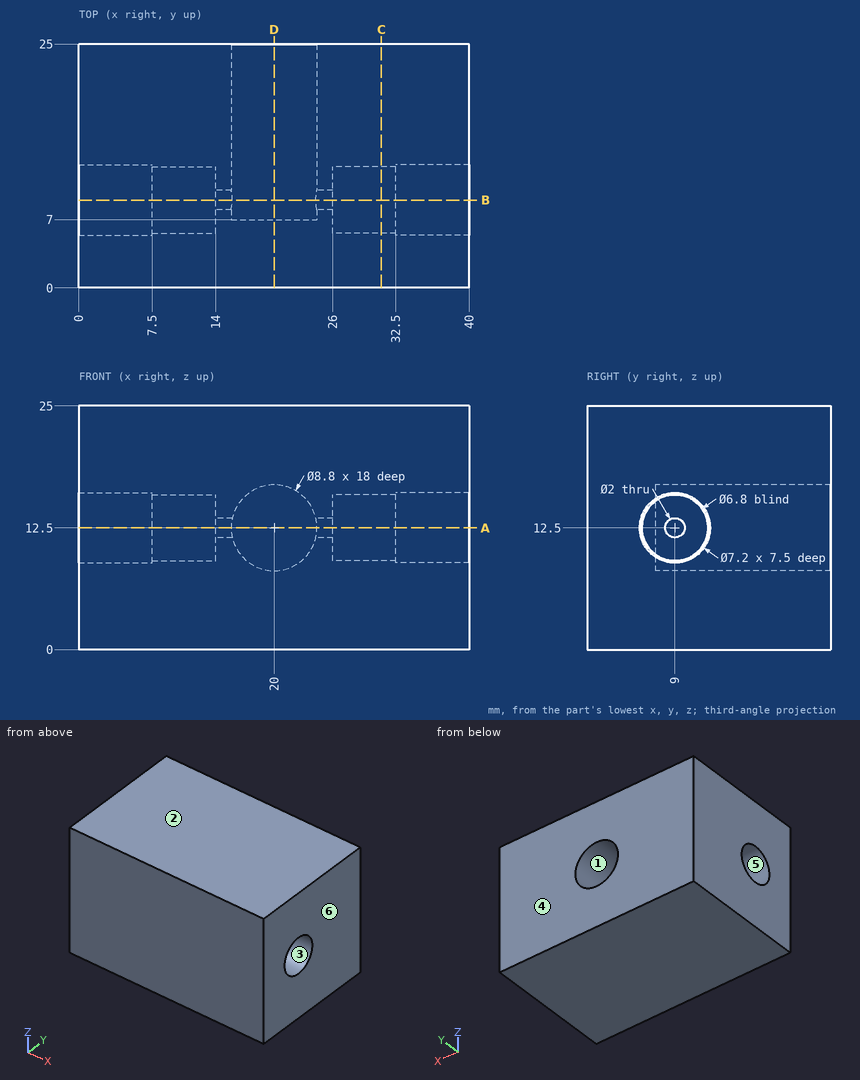
Geometry check sheet. Reference: drawing and pictorial views, mm from the part's lowest x, y, z. A direction names the side the tool comes from. Coordinates: 2 decimals unless noted, no trailing zeros. Write each loop counter-clockwise with the first axis right and the second up, starting at its lowest first coordinate (ties: lowest second). Pieces come first, ordered by that corner, then holes. Notation, with made-up numbers: M 11,22.25 L 61,22.25 A13 cw 61,33.25 Z; hole C 67.25,-34 d7. An arc over 180 degrees is marked long. Use one line per item in the form item = value.
Item 1: Set-up check for the marked faces 1, 2 and 3: record each of +Z, -Z, +X, -X, +Y, -Y from which the full face is reachable in a straight line by a thin tool's end or side.
Answer below:
face_1 = +Y
face_2 = +Z, +X, -X, +Y, -Y
face_3 = +X
Item 2: Gauge pin test, flat ends, axial feed: pin 1 Ø3.5 at (y, z) = (10, 11) entering from +X; pin 2 Ø2 at (y, z) = (10.5, 14) entering from +X; pin 3 Ø2 at (y, z) = (8, 14) entering from -X; pin 4 Ø1.8 at (y, z) = (9, 12.5) entering from +X. Record the tip position at first contact, or that the pin passes through.
Answer below:
pin_1 = 32.5
pin_2 = 26
pin_3 = 14
pin_4 = through
Item 3: Sectioned sample at A-A, the plane z = 12.5. State how many separate pieces and enclosed holes the cut face has, and give its area (3 significant figures).
Answer below:
separate_pieces = 3
enclosed_holes = 0
area = 639 mm^2
Item 4: Release check for a two-part mould opening along Y. For the marked faces 4, 5 and 6 record: pulls with the +Y half, pulls with the -Y half, needs draft (parallel to the pull), parting line crosses it, or undercut.
Answer below:
face_4 = pulls with the +Y half
face_5 = undercut
face_6 = needs draft
Item 5: Sectioned sample at D-D, the plane x = 20. Record the cut outline in (y, z), and give its area (3 significant figures).
Answer below:
outline = M 0,0 L 25,0 L 25,8.1 L 7,8.1 L 7,16.9 L 25,16.9 L 25,25 L 0,25 Z
area = 467 mm^2
Item 6: Material ranges on L1, parallel to Z at x = 10.5, y = 9; L2, parallel to Y at x = 14.6, z = 12.5; L3, parallel to Z at x = 25.45, y = 9, recorded low to high. Write a range as from..to.
Answer below:
L1 = 0..9.1, 15.9..25
L2 = 0..8, 10..25
L3 = 0..11.5, 13.5..25
Item 7: Sectioned sample at B-B, the plane y = 9. Record the cut outline in (x, z), and give its area (3 significant figures).
Answer below:
outline = M 0,0 L 40,0 L 40,8.9 L 32.5,8.9 L 32.5,9.1 L 26,9.1 L 26,11.5 L 24.28,11.5 A4.4 cw 15.72,11.5 L 14,11.5 L 14,9.1 L 7.5,9.1 L 7.5,8.9 L 0,8.9 Z; M 0,16.1 L 7.5,16.1 L 7.5,15.9 L 14,15.9 L 14,13.5 L 15.72,13.5 A4.4 cw 24.28,13.5 L 26,13.5 L 26,15.9 L 32.5,15.9 L 32.5,16.1 L 40,16.1 L 40,25 L 0,25 Z
area = 736 mm^2
Item 8: Sectioned sample at C-C, the plane x = 31. Record the cut outline in (y, z).
Answer below:
outline = M 0,0 L 25,0 L 25,25 L 0,25 Z; hole C 9,12.5 d6.8
